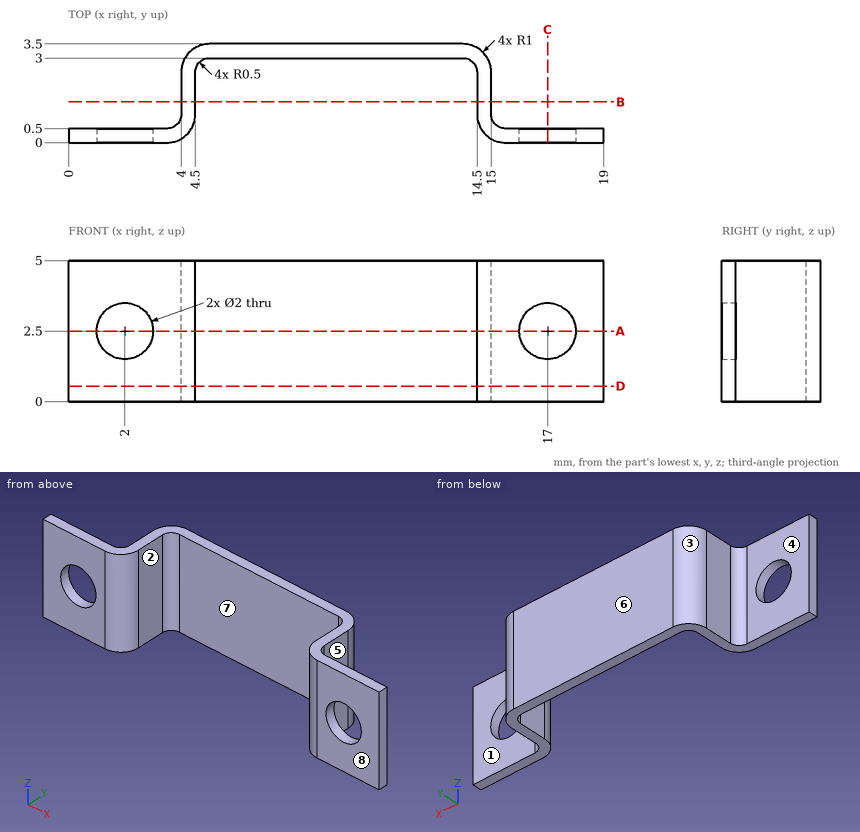
Could you check a few things on this drawing? It's one solid part, dimensions in mm from its lowest x, y, z. A direction names the side the tool comes from. Give positions to 0.01 mm unless a question says otherwise; leave off trailing zeros. Order: outer loops, then holes, each group sorted by start corner. A loop starts at its lowest first (then second) coordinate and runs counter-clockwise, first axis right, second up. Notation, with made-up numbers: (81, 86.5) -> (91, 86.5) arc R25 cw to (91, 124.5) -> close; hole circle Ø4 at (11, 52). An arc over 180 degrees is marked (long way). Use CSV: the item, a comma, the result in double quotes. Start each with the question number.
Item 1: Suppose I cut it at B-B (y = 1.45). List the corners of the cut face in (x, z) for me.
Item 2: I'm going to push flat-ended pins straight in: P1, Ø3, axis at x = 1, z = 3, coming from the +Y side; P2, Ø2.5, axis at x = 17, z = 2.5, coming from the -Y side; P3, Ø1.6, axis at y = 1.5, z = 3, coming from the -X side. Where does each tip first touch, or does it pass through?
Item 3: Suppose I cut it at D-D (z = 0.55). List the corners of the cut face in (x, y) for me.
Item 4: If I drill on probe 1 along Z at (x, y) = (2, 0.3); probe 2 along X at (y, z) = (1.25, 4.45); probe 3 along Y at (x, z) = (16, 2.05), over which ranges is the centre line in solid material (lowest first)? Write a range as [from, to].
Item 5: Suppose I cut it at C-C (x = 17). List the corners of the cut face in (y, z) for me, and give its area (3 significant figures).
Item 6: On a 3-axis mill with a long thin cutter (end or side, diameter ignored), from which of +Z, -Z, +X, -X, +Y, -Y can I reach the whole of each face in a straight line? I mean the marked faces 4, 5, 6, 7 and 8. Say none if no direction works.
Item 7: Suppose I cut it at A-A (z = 2.5). List the corners of the cut face in (x, y) for me, and give its area (3 significant figures).
Item 8: Thinking about a two-plate mould opening in X: for the marked faces 1, 2 and 3, which applies, pulls with the +X half, pulls with the -X half, needs draft (parallel to the pull), parting line crosses it, or undercut?
Answer block:
1,outline,"(4, 0) -> (4.5, 0) -> (4.5, 5) -> (4, 5) -> close; (14.5, 0) -> (15, 0) -> (15, 5) -> (14.5, 5) -> close"
2,P1,"stops at y = 0.5"
2,P2,"stops at y = 0"
2,P3,"stops at x = 3.9"
3,outline,"(0, 0) -> (3.5, 0) arc R1 ccw to (4.5, 1) -> (4.5, 2.5) arc R0.5 cw to (5, 3) -> (14, 3) arc R0.5 cw to (14.5, 2.5) -> (14.5, 1) arc R1 ccw to (15.5, 0) -> (19, 0) -> (19, 0.5) -> (15.5, 0.5) arc R0.5 cw to (15, 1) -> (15, 2.5) arc R1 ccw to (14, 3.5) -> (5, 3.5) arc R1 ccw to (4, 2.5) -> (4, 1) arc R0.5 cw to (3.5, 0.5) -> (0, 0.5) -> close"
4,probe 1,"z = [0, 1.5], [3.5, 5]"
4,probe 2,"x = [4, 4.5], [14.5, 15]"
4,probe 3,"y = [0, 0.5]"
5,outline,"(0, 0) -> (0.5, 0) -> (0.5, 1.5) -> (0, 1.5) -> close; (0, 3.5) -> (0.5, 3.5) -> (0.5, 5) -> (0, 5) -> close"
5,area,"1.50 mm^2"
6,face 4,"+Z, -Z, -X, +Y"
6,face 5,"+Z, -Z, +X, +Y"
6,face 6,"+Z, -Z, +X, -X, +Y"
6,face 7,"+Z, -Z, -Y"
6,face 8,"+Z, -Z, +X, -X, -Y"
7,outline,"(0, 0) -> (1, 0) -> (1, 0.5) -> (0, 0.5) -> close; (3, 0) -> (3.5, 0) arc R1 ccw to (4.5, 1) -> (4.5, 2.5) arc R0.5 cw to (5, 3) -> (14, 3) arc R0.5 cw to (14.5, 2.5) -> (14.5, 1) arc R1 ccw to (15.5, 0) -> (16, 0) -> (16, 0.5) -> (15.5, 0.5) arc R0.5 cw to (15, 1) -> (15, 2.5) arc R1 ccw to (14, 3.5) -> (5, 3.5) arc R1 ccw to (4, 2.5) -> (4, 1) arc R0.5 cw to (3.5, 0.5) -> (3, 0.5) -> close; (18, 0) -> (19, 0) -> (19, 0.5) -> (18, 0.5) -> close"
7,area,"9.86 mm^2"
8,face 1,"needs draft"
8,face 2,"undercut"
8,face 3,"pulls with the -X half"
